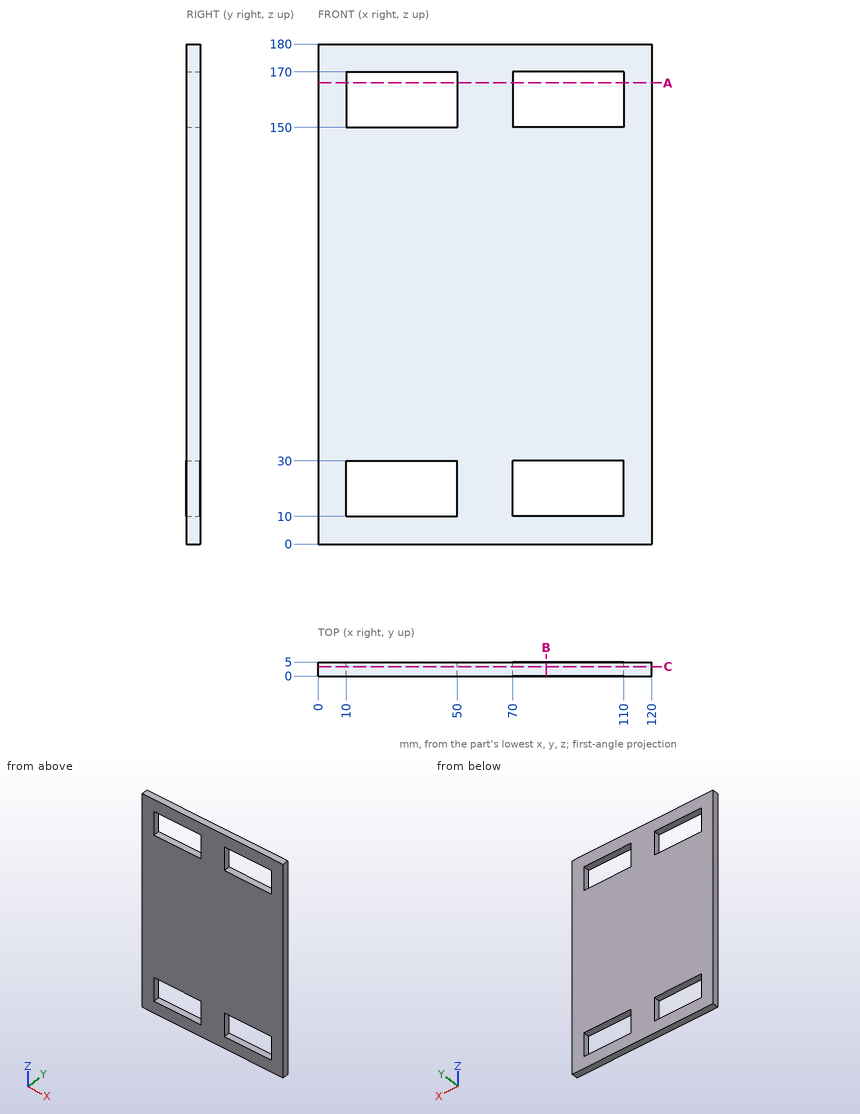
Geometry check sheet. Reference: drawing and pictorial views, mm from the part's lowest x, y, z. Give positions to 0.01 mm unless a question says otherwise; leave off trailing zeros. Loops run counter-clockwise (first coordinate to the right, second up) from the corner with the lowest first, then second, coordinate; pieces in that order, holes last. Notation, with made-up numbers: M 88.25,51.5 L 93.25,51.5 A20 cw 93.25,74.5 Z; hole C 82,-22.75 d5. An arc over 180 degrees is marked long. Use a Markdown table: item, result. Add a question column.
Q1. Sectioned sample at A-A, the plane z = 166. Record the cut outline in (x, y), then the cut area to 3 significant figures.
Q2. Scan lines: line 1 along Z through (x, y) = (24, 1.05); line 2 along X through (y, z) = (4.05, 154). Record each from-to range of solid material in increasing order. Write a range as [from, to].
Q3. Sectioned sample at B-B, the plane x = 82. Record the cut outline in (y, z), then the cut area to 3 significant figures.
Q4. Sectioned sample at C-C, the plane y = 3.4. Record the cut outline in (x, z).
Verdict:
| question | item | result |
|---|---|---|
| 1 | outline | M 0,0 L 10,0 L 10,5 L 0,5 Z; M 50,0 L 70,0 L 70,5 L 50,5 Z; M 110,0 L 120,0 L 120,5 L 110,5 Z |
| 1 | area | 200 mm^2 |
| 2 | line 1 | [0, 10], [30, 150], [170, 180] |
| 2 | line 2 | [0, 10], [50, 70], [110, 120] |
| 3 | outline | M 0,0 L 5,0 L 5,10 L 0,10 Z; M 0,30 L 5,30 L 5,150 L 0,150 Z; M 0,170 L 5,170 L 5,180 L 0,180 Z |
| 3 | area | 700 mm^2 |
| 4 | outline | M 0,0 L 120,0 L 120,180 L 0,180 Z; hole M 10,10 L 50,10 L 50,30 L 10,30 Z; hole M 10,150 L 50,150 L 50,170 L 10,170 Z; hole M 70,10 L 110,10 L 110,30 L 70,30 Z; hole M 70,150 L 110,150 L 110,170 L 70,170 Z |
